The listing builds one solid part. Answer for the finished solid, in the listing's coordinates (mm). Face numbers are marked on the shaded views. A direction names the side the tool comes from. Round coordinates to 2 decimals unless told otherwise and drop trailing zeros. Order: outer loops, then holes, each group sorted by start corner. A loop starts at its lowest first (then second) coordinate and runs counter-clockwise, first axis right, second up. Notation, with made-up numbers: (42.25, 60) -> (92.25, 60) arc R12 ccw to (92.25, 83) -> close; hole circle Ø8 at (82, -16). An arc over 180 degrees is marked (long way). Return JSON: item names as keys, results as strings. Group by question number.
(1) Determine the mould class of the marked faces 3, 4 and 5 for opening direction Z: +Z half, -Z half, draft (parallel to the pull), parting line (faces both ways), or undercut.
(2) The part is cut by section B-B (x = 18). Determine the outline of the cut face in (y, z), plus the area to 3 significant figures.
(3) Each of these flat-tipped pins is pushed along its axis until it touches: pin 1 (1.5 mm diameter, centred on x = 13, z = -8.5, fed in from -Y); pin 2 (1.5 mm diameter, centred on x = -10.5, z = -18.5, fed in from +Y); pin 3 (1.6 mm diameter, centred on x = -9, y = 1, fed in from +Z). Where does it stop, or does it pass through?
(4) Consider line 1 (X direction, y = -6.25, z = -24.5); line 2 (Y direction, x = 6, z = -7.5); line 3 (Z direction, x = -11, y = 0.75). Determine where each line is inside the solid, lowest interval first. Write a range as [from, to].
(5) Which of the six approach directions +Z, -Z, +X, -X, +Y, -Y give full straight-line access (tool end or side, diameter ignored) to the marked faces 1 and 2?
(6) The part is cut by section A-A (y = -4). Determine the outline of the cut face in (x, z), plus the area to 3 significant figures.
(7) The part is cut by section C-C (y = 6). Determine the outline of the cut face in (x, z) (3 decimals), plus the area to 3 significant figures.
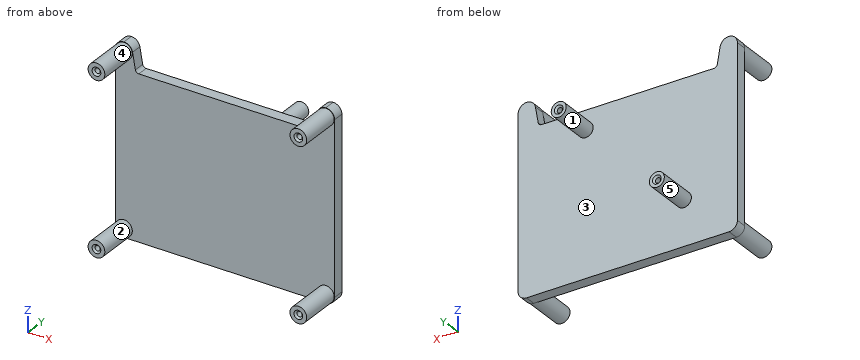
from build123d import *

# Parameters (mm, degrees)
BOSS_EXTRUDE1_DEPTH = 3.2
SKETCH2_R           = 2.4
SKETCH2_R_2         = 0.75
BOSS_EXTRUDE2_DEPTH = 12
SKETCH3_R           = 2.15
SKETCH3_R_2         = 0.75
BOSS_EXTRUDE3_DEPTH = 11.8
CHAMFER1_SIZE       = 0.5
CHAMFER2_SIZE       = 1.9
CHAMFER2_SIZE_2     = 10.775435457
FILLET1_R           = 2.4
FILLET2_R           = 2.501224
FILLET3_R           = 2.501224
FILLET4_R           = 1


# Some blends are built 0.0001 mm under size
with BuildPart() as part:
    # Sketch1 → Boss-Extrude1 (new body)
    with BuildSketch(Plane(origin=(0, 0, 0), x_dir=(1, 0, 0), z_dir=(0, 1, 0))):
        Polygon((31.5, 27), (-31.5, 27), (-31.5, -27), (-25, -27), (-25, -19.5), (25, -19.5), (25, -27), (31.5, -27), align=None)
    extrude(amount=BOSS_EXTRUDE1_DEPTH)

    # Sketch2 → Boss-Extrude2 (add)
    # profile 1 of 4: a face of its own
    with BuildSketch(Plane.XZ):
        with Locations(Location((-29, -24.5, 0), (0, 0, 90))):
            Circle(SKETCH2_R)
        with Locations(Location((-29, -24.5, 0), (0, 0, 270))):
            Circle(SKETCH2_R_2, mode=Mode.SUBTRACT)
    # profile 2 of 4: a face of its own
    with BuildSketch(Plane.XZ):
        with Locations(Location((29, -24.5, 0), (0, 0, 90))):
            Circle(SKETCH2_R)
        with Locations(Location((29, -24.5, 0), (0, 0, 90))):
            Circle(SKETCH2_R_2, mode=Mode.SUBTRACT)
    # profile 3 of 4: a face of its own
    with BuildSketch(Plane.XZ):
        with Locations(Location((29, 24.5, 0), (0, 0, 90))):
            Circle(SKETCH2_R)
        with Locations(Location((29, 24.5, 0), (0, 0, 270))):
            Circle(SKETCH2_R_2, mode=Mode.SUBTRACT)
    # profile 4 of 4: a face of its own
    with BuildSketch(Plane.XZ):
        with Locations(Location((-29, 24.5, 0), (0, 0, 90))):
            Circle(SKETCH2_R)
        with Locations(Location((-29, 24.5, 0), (0, 0, 90))):
            Circle(SKETCH2_R_2, mode=Mode.SUBTRACT)
    extrude(amount=BOSS_EXTRUDE2_DEPTH)

    # Sketch3 → Boss-Extrude3 (add)
    # profile 1 of 2: a face of its own
    with BuildSketch(Plane(origin=(0, 3.2, 0), x_dir=(1, 0, 0), z_dir=(0, 1, 0))):
        with Locations(Location((-16.125, 14.125, 0), (0, 0, 270))):
            Circle(SKETCH3_R)
        with Locations(Location((-16.125, 14.125, 0), (0, 0, 270))):
            Circle(SKETCH3_R_2, mode=Mode.SUBTRACT)
    # profile 2 of 2: a face of its own
    with BuildSketch(Plane(origin=(0, 3.2, 0), x_dir=(1, 0, 0), z_dir=(0, 1, 0))):
        with Locations(Location((12.075, -14.075, 0), (0, 0, 270))):
            Circle(SKETCH3_R)
        with Locations(Location((12.075, -14.075, 0), (0, 0, 270))):
            Circle(SKETCH3_R_2, mode=Mode.SUBTRACT)
    extrude(amount=BOSS_EXTRUDE3_DEPTH)

    # Chamfer1
    chamfer1_edges = [part.edges().sort_by_distance(p)[0] for p in [
        (-29, -12, -23.75),
        (29, -12, -25.25),
        (29, -12, 25.25),
        (-29, -12, 23.75),
        (-16.125, 15, -14.875),
        (12.075, 15, 13.325),
    ]]
    chamfer(chamfer1_edges, length=CHAMFER1_SIZE)

    # Chamfer2
    # the kernel refuses this chamfer: 10.775435457, 1.9 mm, written as the material it takes off along each edge
    with BuildSketch(Plane(origin=(25, -28.000387084, 27), x_dir=(0.9776715712462577, 0, 0.2101387607674357), z_dir=(0, 1, 0))) as chamfer2_piece_1_section:
        Polygon((CHAMFER2_SIZE * 0.977671571246, CHAMFER2_SIZE * 0.210138760767), (-CHAMFER2_SIZE_2 * 0.210138760773, CHAMFER2_SIZE_2 * 0.977671571271), (0, 0), align=None)
    chamfer2_piece_1 = extrude(amount=59.200774168, mode=Mode.PRIVATE)
    chamfer2_piece_1 = split(chamfer2_piece_1, bisect_by=Plane(origin=(25.592384699, 1.6, 19.5), z_dir=(0, 0, 1)), keep=Keep.TOP, mode=Mode.PRIVATE)
    add(chamfer2_piece_1, mode=Mode.SUBTRACT)
    with BuildSketch(Plane(origin=(-25, -28.000387084, 27), x_dir=(0.006682531656101439, 0, -0.9999776716360547), z_dir=(0, 1, 0))) as chamfer2_piece_2_section:
        Polygon((CHAMFER2_SIZE_2 * 0.999977671661, CHAMFER2_SIZE_2 * 0.00668253165627), (-CHAMFER2_SIZE * 0.0066825316561, CHAMFER2_SIZE * 0.999977671636), (0, 0), align=None)
    chamfer2_piece_2 = extrude(amount=59.200774168, mode=Mode.PRIVATE)
    chamfer2_piece_2 = split(chamfer2_piece_2, bisect_by=Plane(origin=(-25.592384699, 1.6, 19.5), z_dir=(0, 0, 1)), keep=Keep.TOP, mode=Mode.PRIVATE)
    add(chamfer2_piece_2, mode=Mode.SUBTRACT)

    # Fillet1
    fillet1_edges = [part.edges().sort_by_distance(p)[0] for p in [
        (-31.5, 1.6, -27),
        (31.5, 1.6, -27),
    ]]
    fillet(fillet1_edges, radius=FILLET1_R)

    # Fillet2
    fillet2_edges = [part.edges().sort_by_distance(p)[0] for p in [
        (31.5, 1.6, 27),
        (26.9, 1.6, 27),
    ]]
    fillet(fillet2_edges, radius=FILLET2_R - 0.0001)  # a hair under: the kernel refuses the full size

    # Fillet3
    fillet3_edges = [part.edges().sort_by_distance(p)[0] for p in [
        (-31.5, 1.6, 27),
        (-26.9, 1.6, 27),
    ]]
    fillet(fillet3_edges, radius=FILLET3_R - 0.0001)  # a hair under: the kernel refuses the full size

    # Fillet4
    fillet4_edges = [part.edges().sort_by_distance(p)[0] for p in [
        (25.577547645, 1.6, 19.5),
        (-25.577547645, 1.6, 19.5),
    ]]
    fillet(fillet4_edges, radius=FILLET4_R)


solid = part.part
Answer below:
{
 "1": {"face 3": "draft", "face 4": "undercut", "face 5": "parting line"},
 "2": {"outline": "(0, -27) -> (3.2, -27) -> (3.2, 19.5) -> (0, 19.5) -> close", "area": "149 mm²"},
 "3": {"pin 1": "stops at y = 0", "pin 2": "stops at y = 3.2", "pin 3": "stops at z = 19.5"},
 "4": {"line 1": "x = [-31.4, -29.75], [-28.25, -26.6], [26.6, 28.25], [29.75, 31.4]", "line 2": "y = [0, 3.2]", "line 3": "z = [-27, 19.5]"},
 "5": {"face 1": "+Y", "face 2": "-Y"},
 "6": {"outline": "circle Ø4.8 at (-29, -24.5); circle Ø4.8 at (-29, 24.5); circle Ø4.8 at (29, -24.5); circle Ø4.8 at (29, 24.5); hole circle Ø1.5 at (-29, -24.5); hole circle Ø1.5 at (-29, 24.5); hole circle Ø1.5 at (29, -24.5); hole circle Ø1.5 at (29, 24.5)", "area": "65.3 mm²"},
 "7": {"outline": "circle Ø4.3 at (-16.125, -14.125); circle Ø4.3 at (12.075, 14.075); hole circle Ø1.5 at (-16.125, -14.125); hole circle Ø1.5 at (12.075, 14.075)", "area": "25.5 mm²"}
}
